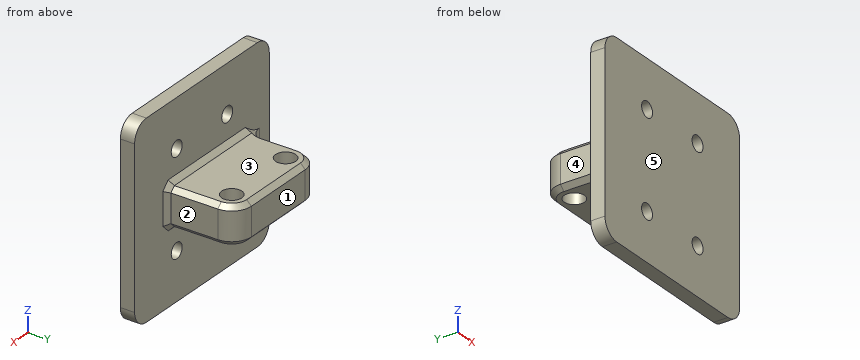
from build123d import *

# Parameters (mm, degrees)
SKETCH1_W           = 40
SKETCH1_H           = 40
BOSS_EXTRUDE1_DEPTH = 3
FILLET1_R           = 3.5
SKETCH2_R           = 2.125
BOSS_EXTRUDE2_DEPTH = 4
FILLET2_R           = 3.5
CHAMFER1_SIZE       = 1
CHAMFER2_SIZE       = 1
SKETCH4_R           = 1.625
CUT_EXTRUDE4_DEPTH  = 10


with BuildPart() as part:
    # Sketch1 → Boss-Extrude1 (new body)
    with BuildSketch(Plane(origin=(0, 0, 0), x_dir=(1, 0, 0), z_dir=(0, 1, 0))):
        Rectangle(SKETCH1_W, SKETCH1_H)
    extrude(amount=BOSS_EXTRUDE1_DEPTH)

    # Fillet1
    fillet1_edges = [part.edges().sort_by_distance(p)[0] for p in [
        (-20, 1.5, 20),
        (-20, 1.5, -20),
        (20, 1.5, -20),
        (20, 1.5, 20),
    ]]
    fillet(fillet1_edges, radius=FILLET1_R)

    # Sketch2 → Boss-Extrude2 (add, symmetric)
    with BuildSketch(Plane.XY):
        with BuildLine():
            Line((-1.5, 0), (10.625, 0))
            Line((10.625, 0), (10.625, 13.875))
            ThreePointArc((10.625, 13.875), (9.416815472, 16.791815472), (6.5, 18))
            Line((6.5, 18), (-9.5, 18))
            ThreePointArc((-9.5, 18), (-12.416815472, 16.791815472), (-13.625, 13.875))
            Line((-13.625, 13.875), (-13.625, 0))
            Line((-13.625, 0), (-1.5, 0))
        make_face()
        with Locations((-9.5, 13.875)):
            Circle(SKETCH2_R, mode=Mode.SUBTRACT)
        with Locations((6.5, 13.875)):
            Circle(SKETCH2_R, mode=Mode.SUBTRACT)
    extrude(amount=BOSS_EXTRUDE2_DEPTH, both=True)

    # Fillet2
    fillet2_edges = [part.edges().sort_by_distance(p)[0] for p in [
        (-13.625, 3, 0),
    ]]
    fillet(fillet2_edges, radius=FILLET2_R)

    # Chamfer1
    # the kernel refuses this chamfer: 1 mm, written as the material it takes off along each edge
    with BuildSketch(Plane(origin=(-17.125, 6.5, -4), x_dir=(-0.6706329473594386, -0.7417893568365567, 0), z_dir=(-0.7417893568365567, 0.6706329473594386, 0))) as chamfer1_piece_1_section:
        Polygon((3.5, CHAMFER1_SIZE), (3.5 + CHAMFER1_SIZE, 0), (3.5, 0), align=None)
    chamfer1_piece_1 = revolve(axis=Axis((-17.125, 6.5, -4), (0, 0, 1)), revolution_arc=132.115934794, mode=Mode.PRIVATE)
    chamfer1_piece_1 = split(chamfer1_piece_1, bisect_by=Plane(origin=(-14.562264523, 3, -3.629385384), z_dir=(0, 1, 0)), keep=Keep.TOP, mode=Mode.PRIVATE)
    add(chamfer1_piece_1, mode=Mode.SUBTRACT)
    with BuildSketch(Plane(origin=(-17.125, 6.5, 4), x_dir=(-0.6706329473594386, -0.7417893568365567, 0), z_dir=(-0.7417893568365567, 0.6706329473594386, 0))) as chamfer1_piece_2_section:
        Polygon((3.5, -CHAMFER1_SIZE), (3.5 + CHAMFER1_SIZE, 0), (3.5, 0), align=None)
    chamfer1_piece_2 = revolve(axis=Axis((-17.125, 6.5, 4), (0, 0, 1)), revolution_arc=132.115934794, mode=Mode.PRIVATE)
    chamfer1_piece_2 = split(chamfer1_piece_2, bisect_by=Plane(origin=(-14.562264523, 3, 3.629385384), z_dir=(0, 1, 0)), keep=Keep.TOP, mode=Mode.PRIVATE)
    add(chamfer1_piece_2, mode=Mode.SUBTRACT)
    with BuildSketch(Plane(origin=(10.625, 3, 4), x_dir=(-0.9996219169112968, 0, 0.02749587661058651), z_dir=(0, 1, 0)), Plane(origin=(10.625, 3, -4), x_dir=(0.027495876610585623, 0, 0.9996219169112968), z_dir=(0, 1, 0))) as chamfer1_piece_3:
        Polygon((CHAMFER1_SIZE * 0.999621916911, -CHAMFER1_SIZE * 0.0274958766106), (-CHAMFER1_SIZE * 0.0274958766106, -CHAMFER1_SIZE * 0.999621916911), (0, 0), align=None)
    extrude(amount=10.875, mode=Mode.SUBTRACT)
    with BuildSketch(Plane(origin=(6.5, 13.875, 4), x_dir=(1, 0, 0), z_dir=(0, -1, 0))) as chamfer1_piece_4:
        Polygon((4.125, -CHAMFER1_SIZE), (4.125 - CHAMFER1_SIZE, 0), (4.125, 0), align=None)
    revolve(axis=Axis((6.5, 13.875, 4), (0, 0, 1)), revolution_arc=90, mode=Mode.SUBTRACT)
    with BuildSketch(Plane(origin=(6.5, 18, 4), x_dir=(0, 0.027495876610585623, -0.9996219169112968), z_dir=(-1, 0, 0))) as chamfer1_piece_5:
        Polygon((CHAMFER1_SIZE * 0.999621916911, CHAMFER1_SIZE * 0.0274958766106), (-CHAMFER1_SIZE * 0.0274958766106, CHAMFER1_SIZE * 0.999621916911), (0, 0), align=None)
    extrude(amount=16, mode=Mode.SUBTRACT)
    with BuildSketch(Plane(origin=(-9.5, 13.875, 4), x_dir=(0, 1, 0), z_dir=(1, 0, 0))) as chamfer1_piece_6:
        Polygon((4.125, -CHAMFER1_SIZE), (4.125 - CHAMFER1_SIZE, 0), (4.125, 0), align=None)
    revolve(axis=Axis((-9.5, 13.875, 4), (0, 0, 1)), revolution_arc=90, mode=Mode.SUBTRACT)
    with BuildSketch(Plane(origin=(-13.625, 13.875, 4), x_dir=(-0.027495876610585623, 0, -0.9996219169112968), z_dir=(0, -1, 0))) as chamfer1_piece_7:
        Polygon((CHAMFER1_SIZE * 0.999621916911, CHAMFER1_SIZE * 0.0274958766106), (-CHAMFER1_SIZE * 0.0274958766106, CHAMFER1_SIZE * 0.999621916911), (0, 0), align=None)
    extrude(amount=7.375, mode=Mode.SUBTRACT)
    with BuildSketch(Plane(origin=(6.5, 13.875, -4), x_dir=(1, 0, 0), z_dir=(0, -1, 0))) as chamfer1_piece_8:
        Polygon((4.125, CHAMFER1_SIZE), (4.125 - CHAMFER1_SIZE, 0), (4.125, 0), align=None)
    revolve(axis=Axis((6.5, 13.875, -4), (0, 0, 1)), revolution_arc=90, mode=Mode.SUBTRACT)
    with BuildSketch(Plane(origin=(6.5, 18, -4), x_dir=(0, 0.027495876610585623, 0.9996219169112968), z_dir=(-1, 0, 0))) as chamfer1_piece_9:
        Polygon((CHAMFER1_SIZE * 0.999621916911, -CHAMFER1_SIZE * 0.0274958766106), (-CHAMFER1_SIZE * 0.0274958766106, -CHAMFER1_SIZE * 0.999621916911), (0, 0), align=None)
    extrude(amount=16, mode=Mode.SUBTRACT)
    with BuildSketch(Plane(origin=(-9.5, 13.875, -4), x_dir=(0, 1, 0), z_dir=(1, 0, 0))) as chamfer1_piece_10:
        Polygon((4.125, CHAMFER1_SIZE), (4.125 - CHAMFER1_SIZE, 0), (4.125, 0), align=None)
    revolve(axis=Axis((-9.5, 13.875, -4), (0, 0, 1)), revolution_arc=90, mode=Mode.SUBTRACT)
    with BuildSketch(Plane(origin=(-13.625, 13.875, -4), x_dir=(-0.027495876610585623, 0, 0.9996219169112968), z_dir=(0, -1, 0))) as chamfer1_piece_11:
        Polygon((CHAMFER1_SIZE * 0.999621916911, -CHAMFER1_SIZE * 0.0274958766106), (-CHAMFER1_SIZE * 0.0274958766106, -CHAMFER1_SIZE * 0.999621916911), (0, 0), align=None)
    extrude(amount=7.375, mode=Mode.SUBTRACT)

    # Chamfer2
    chamfer2_edges = [part.edges().sort_by_distance(p)[0] for p in [
        (-2.335786438, 3, -4),
        (10.625, 3, 0),
        (-2.335786438, 3, 4),
        (10.125, 3, -3.5),
        (10.125, 3, 3.5),
    ]]
    chamfer(chamfer2_edges, length=CHAMFER2_SIZE)

    # Sketch4 → Cut-Extrude4 (cut)
    with BuildSketch(Plane(origin=(0, 0, 0), x_dir=(1, 0, 0), z_dir=(0, 1, 0))):
        with Locations(Location((-7.5, 10, 0), (0, 0, 270))):
            Circle(SKETCH4_R)
        with Locations(Location((7.5, 10, 0), (0, 0, 270))):
            Circle(SKETCH4_R)
        with Locations(Location((7.5, -10, 0), (0, 0, 270))):
            Circle(SKETCH4_R)
        with Locations(Location((-7.5, -10, 0), (0, 0, 270))):
            Circle(SKETCH4_R)
    extrude(amount=CUT_EXTRUDE4_DEPTH, mode=Mode.SUBTRACT)


solid = part.part
Input: part model. Units: mm. Frame: model coordinates. Face numbers are marked on the shaded views. A direction names the side the tool comes from. Coordinates: 2 decimals unless noted, no trailing zeros. Order: outer loops, then holes, each group sorted by start corner. A loop starts at its lowest first (then second) coordinate and runs counter-clockwise, first axis right, second up. Notation, with made-up numbers: M 81,22.5 L 109,22.5 A25 ccw 109,51.5 Z; hole C 12.5,20.5 d3. An arc over 180 degrees is marked long. Answer in a Markdown table with one row per item.
(1) Section query A-A, the plane z = 10. Output: boundary loops of the cut face in (x, y) (3 decimals), plus the area to 4 significant figures.
Numbers:
| item | result |
|---|---|
| outline | M -20,0 L -9.125,0 L -9.125,3 L -20,3 Z; M -5.875,0 L 5.875,0 L 5.875,3 L -5.875,3 Z; M 9.125,0 L 20,0 L 20,3 L 9.125,3 Z |
| area | 100.5 mm^2 |
(2) Access query for the marked faces 1, 2, 3, 4 and 5. Directions: +Z, -Z, +X, -X, +Y, -Y. A direction counts if a zero-diameter tool reaches every point of the face in a straight line with its end or side. Return the directions, or none.
Numbers:
| item | result |
|---|---|
| face 1 | +Z, -Z, +X, -X, +Y |
| face 2 | +Z, -Z, +X, +Y |
| face 3 | +Z, +X, -X, +Y |
| face 4 | +Z, -Z, -X, +Y |
| face 5 | +Z, -Z, +X, -X, -Y |
(3) Section query D-D, the plane x = -2.5. Output: boundary loops of the cut face in (y, z), plus the area to 3 significant figures.
Numbers:
| item | result |
|---|---|
| outline | M 0,-20 L 3,-20 L 3,-5 L 4,-4 L 17,-4 L 18,-3 L 18,3 L 17,4 L 4,4 L 3,5 L 3,20 L 0,20 Z |
| area | 240 mm^2 |
(4) Contact query for flat-ended pins moving along their axis: pin 1 Ø1 at (x, z) = (12, 6) entering from +Y; pin 2 Ø4 at (x, z) = (-7.5, -10) entering from -Y; pin 3 Ø10.5 at (x, y) = (3, 9.5) entering from +Z; pin 4 Ø6.5 at (y, z) = (12, -0.5) entering from -X (3 decimals). Output: stop coordinate, or through.
Numbers:
| item | result |
|---|---|
| pin 1 | stops at y = 3 |
| pin 2 | stops at y = 0 |
| pin 3 | stops at z = 4 |
| pin 4 | stops at x = -13.625 |
(5) Material intervals for line 1 (X direction, y = 1.35, z = 10) (3 decimals); line 2 (Z direction, x = -7.5, y = 2.15) (3 decimals); line 3 (Y direction, x = 2, z = 6), sorted ascending. Write a range as [from, to].
Numbers:
| item | result |
|---|---|
| line 1 | x = [-20, -9.125], [-5.875, 5.875], [9.125, 20] |
| line 2 | z = [-20, -11.625], [-8.375, 8.375], [11.625, 20] |
| line 3 | y = [0, 3] |
(6) Section query C-C, the plane y = 11. Output: boundary loops of the cut face in (x, z) (3 decimals).
Numbers:
| item | result |
|---|---|
| outline | M -13.625,-3 L -12.625,-4 L 9.625,-4 L 10.625,-3 L 10.625,3 L 9.625,4 L -12.625,4 L -13.625,3 Z |
(7) Section query B-B, the plane z = 2. Output: boundary loops of the cut face in (x, y) (3 decimals), plus the area to 3 significant figures.
Numbers:
| item | result |
|---|---|
| outline | M -20,0 L 20,0 L 20,3 L 11.625,3 L 10.625,4 L 10.625,13.875 A4.125 ccw 6.5,18 L -9.5,18 A4.125 ccw -13.625,13.875 L -13.625,6.5 A3.5 cw -17.125,3 L -20,3 Z; hole C -9.5,13.875 d4.25; hole C 6.5,13.875 d4.25 |
| area | 451 mm^2 |
